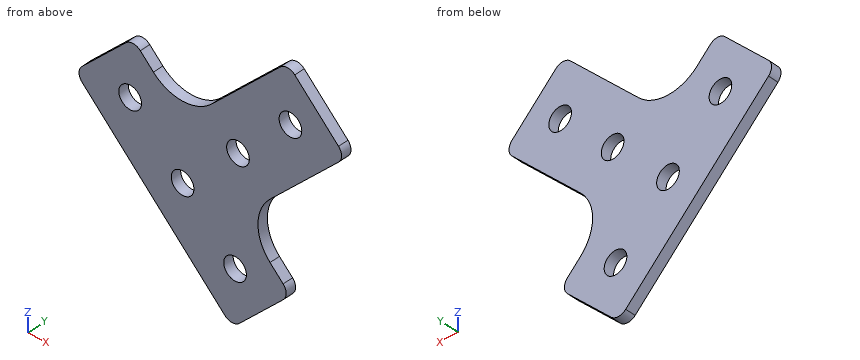
from build123d import *

# Parameters (mm, degrees)
BOSS_EXTRUDE1_DEPTH = 3.175
SKETCH2_R           = 3.4925
CUT_EXTRUDE2_DEPTH  = 3.175
LPATTERN5_COUNT     = 3
LPATTERN5_PITCH     = 22.86
SKETCH7_R           = 3.4925
CUT_EXTRUDE3_DEPTH  = 3.175
LPATTERN6_COUNT     = 2
LPATTERN6_PITCH     = 22.86
SKETCH8_R           = 3.4925
CUT_EXTRUDE4_DEPTH  = 85.115331985
FILLET3_R           = 12.7
FILLET4_R           = 3.175


with BuildPart() as part:
    # Sketch1 → Boss-Extrude1 (new body)
    with BuildSketch(Plane(origin=(0, 0, 0), x_dir=(1, 0, 0), z_dir=(0, 1, 0))):
        Polygon((-17.960512242, 17.960512242), (0, 35.921024484), (17.960512242, 17.960512242), (50.289434278, -14.368409794), (32.328922036, -32.328922036), (0, 0), (-31.430896424, -31.430896424), (-49.391408666, -13.470384182), align=None)
    extrude(amount=BOSS_EXTRUDE1_DEPTH)

    # Sketch2 → Cut-Extrude2 (cut)
    with BuildSketch(Plane(origin=(0, 3.175, 0), x_dir=(1, 0, 0), z_dir=(0, 1, 0))):
        with Locations(Location((-32.328922036, -14.368409794, 0), (0, 0, 270))):
            Circle(SKETCH2_R)
    cut_extrude2 = extrude(amount=-CUT_EXTRUDE2_DEPTH, mode=Mode.SUBTRACT)

    # LPattern5: Cut-Extrude2 ×3
    with Locations(*[Vector(0.7071067811865467, 0, -0.7071067811865485) * (i * LPATTERN5_PITCH) for i in range(1, LPATTERN5_COUNT)]):
        add(cut_extrude2, mode=Mode.SUBTRACT)

    # Sketch7 → Cut-Extrude3 (cut)
    with BuildSketch(Plane(origin=(0, 3.175, 0), x_dir=(1, 0, 0), z_dir=(0, 1, 0))):
        with Locations(Location((33.226947648, -15.266435406, 0), (0, 0, 270))):
            Circle(SKETCH7_R)
    cut_extrude3 = extrude(amount=-CUT_EXTRUDE3_DEPTH, mode=Mode.SUBTRACT)

    # LPattern6: Cut-Extrude3 ×2
    with Locations(*[Vector(-0.7071067811865457, 0, -0.7071067811865493) * (i * LPATTERN6_PITCH) for i in range(1, LPATTERN6_COUNT)]):
        add(cut_extrude3, mode=Mode.SUBTRACT)

    # Mirror2: part across plane


with BuildPart() as part_1:
    add(part.part)
    add(part.part.mirror(Plane(origin=(8.980256121, 0, -8.980256121), x_dir=(0.7071067811865464, 0, 0.7071067811865487), z_dir=(-0.7071067811865489, 0, 0.7071067811865462))))

    # Sketch8 → Cut-Extrude4 (cut, through all)
    # profile 1 of 2: a face of its own
    with BuildSketch(Plane(origin=(0, 3.175, 0), x_dir=(1, 0, 0), z_dir=(0, 1, 0))):
        Polygon((-15.266435406, -15.266435406), (-33.226947648, 2.694076836), (-49.391408666, -13.470384182), (-31.430896424, -31.430896424), align=None)
        with Locations((-32.328922036, -14.368409794)):
            Circle(SKETCH8_R, mode=Mode.SUBTRACT)
    # profile 2 of 2: a face of its own
    with BuildSketch(Plane(origin=(0, 3.175, 0), x_dir=(1, 0, 0), z_dir=(0, 1, 0))):
        Polygon((33.226947648, 33.226947648), (49.391408666, 49.391408666), (31.430896424, 67.351920908), (15.266435406, 51.18745989), align=None)
        with Locations((32.328922036, 50.289434278)):
            Circle(SKETCH8_R, mode=Mode.SUBTRACT)
    extrude(amount=-CUT_EXTRUDE4_DEPTH, mode=Mode.SUBTRACT)

    # Fillet3
    fillet3_edges = [part_1.edges().sort_by_distance(p)[0] for p in [
        (0, 1.5875, 0),
        (17.960512242, 1.5875, -17.960512242),
    ]]
    fillet(fillet3_edges, radius=FILLET3_R)

    # Fillet4
    fillet4_edges = [part_1.edges().sort_by_distance(p)[0] for p in [
        (15.266435406, 1.5875, -51.18745989),
        (33.226947648, 1.5875, -33.226947648),
        (50.289434278, 1.5875, 14.368409794),
        (32.328922036, 1.5875, 32.328922036),
        (-33.226947648, 1.5875, -2.694076836),
        (-15.266435406, 1.5875, 15.266435406),
    ]]
    fillet(fillet4_edges, radius=FILLET4_R)


solid = part_1.part
Input: part model. Units: mm. Frame: model coordinates. Give positions to 0.01 mm unless a question says otherwise; leave off trailing zeros. Order: outer loops, then holes, each group sorted by start corner. A loop starts at its lowest first (then second) coordinate and runs counter-clockwise, first axis right, second up. Notation, with made-up numbers: (0.25, -20) -> (58.25, -20) arc R20 ccw to (58.25, -5) -> close; hole circle Ø6 at (58, 73.25). An arc over 180 degrees is marked (long way). Use one line per item in the form item = value.
1) Section B-B, the plane y = 2.6. Count the separate pieces of the cut face and the enclosed holes in it, and give its area (3 significant figures).
Response values:
separate_pieces = 1
enclosed_holes = 5
area = 2,770 mm^2
2) First-contact query: pin 1 Ø1.5 at (x, y) = (11.5, 2.5) entering from +Z; pin 2 Ø1.5 at (x, y) = (24, 0.5) entering from -Z. Flat tips, straight axial feed; report the tip coordinate or a pass-through.
Response values:
pin_1 = 12.25
pin_2 = -43.2
3) Section C-C, the plane x = 24.5. Return loops of the section in (y, z) (3 decimals), and give its area (3 significant figures).
Response values:
outline = (0, -41.954) -> (3.175, -41.954) -> (3.175, -23.515) -> (0, -23.515) -> close; (0, -12.406) -> (3.175, -12.406) -> (3.175, 24.5) -> (0, 24.5) -> close
area = 176 mm^2
4) Section D-D, the plane z = -40.5. Return loops of the section in (x, y) (3 decimals), and give its area (3 significant figures).
Response values:
outline = (4.579, 0) -> (25.954, 0) -> (25.954, 3.175) -> (4.579, 3.175) -> close
area = 67.9 mm^2
5) Section A-A, the plane x = 0. Return loops of the section in (y, z) (3 decimals).
Response values:
outline = (0, -35.921) -> (3.175, -35.921) -> (3.175, -21.453) -> (0, -21.453) -> close; (0, -14.468) -> (3.175, -14.468) -> (3.175, 5.261) -> (0, 5.261) -> close
6) Line query: probe 1 along X at (y, z) = (2.4, -4); probe 2 along X at (y, z) = (2.4, -9); probe 3 along Z at (x, y) = (33, 0.7). Output: solid intervals per line, ascending.
Response values:
probe_1 = -31.63 to -18.87, -13.46 to 15.46, 18.67 to 31.92
probe_2 = -26.92 to 26.92
probe_3 = -2.92 to 11.78, 18.75 to 30.94
